from build123d import *

# Parameters (mm, degrees)
F1_DEPTH  = 64
F3_D      = 12
F5_DEPTH  = 21
F7_DEPTH  = 8
F9_DEPTH  = 21
F11_DEPTH = 8
F13_DEPTH = 25
F14_D     = 8.5


with BuildPart() as f1:
    # F0 (on Top) → F1 (new body)
    with BuildSketch(Plane.XY):
        Polygon((-65, 0), (-1.9, 0), (0, -2), (0, 20), (-70.3589838486, 20), align=None)
    extrude(amount=F1_DEPTH)

    # F3 (through all)
    with Locations(Plane(origin=(-60.645825623, -16.25, 0), x_dir=(0.2588190451, -0.9659258263, 0), z_dir=(-0.9659258263, -0.2588190451, 0))):
        with Locations((-24.5287615399, 48), (-24.5287615399, 16)):
            Hole(F3_D / 2)

    # F4 (on face) → F5 (join)
    with BuildSketch(Plane(origin=(0, 0, 0), x_dir=(1, 0, 0), z_dir=(0, 0, -1))):
        Polygon((-35, -20), (0, -20), (0, 0), (-1.9, 0), (-35, 0), align=None)
        Polygon((-1.9, 0), (0, 0), (0, 2), align=None)
    extrude(amount=F5_DEPTH)

    # F6 (on face) → F7 (cut)
    with BuildSketch(Plane(origin=(0, 20, 0), x_dir=(-1, 0, 0), z_dir=(0, 1, 0))):
        Polygon((25.897114317, -17.25), (29.7942286341, -10.5), (22, -10.5), (22, -17.25), align=None)
        Polygon((22, -10.5), (29.7942286341, -10.5), (25.897114317, -3.75), (18.102885683, -3.75), (14.2057713659, -10.5), align=None)
        Polygon((22, -17.25), (22, -10.5), (14.2057713659, -10.5), (18.102885683, -17.25), align=None)
    extrude(amount=-F7_DEPTH, mode=Mode.SUBTRACT)

    # F8 (on face) → F9 (join)
    with BuildSketch(Plane.XY.offset(64)):
        Polygon((0, 0), (0, 20), (-35, 20), (-35, 0), (-1.9, 0), align=None)
        Polygon((0, -2), (0, 0), (-1.9, 0), align=None)
    extrude(amount=F9_DEPTH)

    # F10 (on face) → F11 (cut)
    with BuildSketch(Plane(origin=(0, 20, 0), x_dir=(-1, 0, 0), z_dir=(0, 1, 0))):
        Polygon((25.7527767497, 68), (29.5055534995, 74.5), (14.4944465005, 74.5), (18.2472232503, 68), align=None)
        Polygon((14.4944465005, 74.5), (29.5055534995, 74.5), (25.7527767497, 81), (18.2472232503, 81), align=None)
    extrude(amount=-F11_DEPTH, mode=Mode.SUBTRACT)

    # F12 (on face) → F13 (cut)
    with BuildSketch(Plane(origin=(0, 12, 0), x_dir=(-1, 0, 0), z_dir=(0, 1, 0))):
        with BuildLine():
            Line((19.875, 70.8193920339), (24.125, 78.1806079661))
            ThreePointArc((24.125, 78.1806079661), (18.3193920339, 76.625), (19.875, 70.8193920339))
        make_face()
        with BuildLine():
            ThreePointArc((26.25, 74.5), (25.6806079661, 76.625), (24.125, 78.1806079661))
            Line((24.125, 78.1806079661), (19.875, 70.8193920339))
            ThreePointArc((19.875, 70.8193920339), (24.125, 70.8193920339), (26.25, 74.5))
        make_face()
    extrude(amount=-F13_DEPTH, mode=Mode.SUBTRACT)

    # F14 (through all)
    with Locations(Plane(origin=(0, 20, 0), x_dir=(-1, 0, 0), z_dir=(0, 1, 0))):
        with Locations((22, -10.5)):
            Hole(F14_D / 2)


solid = f1.part
Verification items for the finished model (mm, model axes). A direction names the side the tool comes from. Coordinates: 2 decimals unless noted, no trailing zeros. Order: outer loops, then holes, each group sorted by start corner. A loop starts at its lowest first (then second) coordinate and runs counter-clockwise, first axis right, second up. Notation, with made-up numbers: M 83,26 L 91,26 A20 ccw 91,43 Z; hole C -33.5,-12 d1. An arc over 180 degrees is marked long. One line per item, written item: value. Start each with the question number.
Item 1: Mould release check, pull along Z, two halves, no side actions. Record for faces 4 (the cylindrical face through (-25.37, 5.92, -13.09)), 5 (the flat face through (-18, 12, 85)), 6 (the flat face through (-35, 10, -10)): pulls with the +Z half, pulls with the -Z half, needs draft (parallel to the pull), parting line crosses it, or undercut.
Item 2: Access from +Z, -Z, +X, -X, +Y, -Y to the whole of each face (thin tool, end or side, straight path). Record for faces 1 (the flat face through (-27, 0, 31)), 2 (the flat face through (-27.6, 16.1, 71.2)), 3 (the cylindrical face through (-39.454, 8.617, 16.264)).
Item 3: Thickness scan on probe 1 along Z at (x, y) = (-22, 4.25); probe 2 along Z at (x, y) = (-21, 12.25); probe 3 along Z at (x, y) = (-27.5, 15.5). Record the ranges inside material, lowest first.
Item 4: Sectioned sample at B-B on x = -22. Give the number of separate pieces and of enclosed holes in the cut face, then the cut area to 3 significant figures.
Item 5: Sectioned sample at A-A on z = 43.5. Record the cut outline in (x, y).
Item 6: Depth check by flat-ended pin: P1, Ø19, axis at x = -46.5, z = 29.5, coming from the -Y side; P2, Ø2, axis at x = -38.5, y = 5, coming from the +Z side; P3, Ø11, axis at x = -22, z = -10.5, coming from the +Y side. Enter the tip coordinate at first touch or a pass-through.
Calculated:
1. face 4: undercut
1. face 5: pulls with the +Z half
1. face 6: needs draft
2. face 1: +Z, -Z, -X, -Y
2. face 2: +Y
2. face 3: none
3. probe 1: -21 to -14.75, -6.25 to 70.25, 78.75 to 85
3. probe 2: -21 to -17.25, -3.75 to 68, 81 to 85
3. probe 3: -21 to -14.47, -6.53 to 10.52, 21.48 to 42.52, 53.48 to 71.03, 77.97 to 85
4. separate pieces: 3
4. enclosed holes: 0
4. area: 1,570 mm^2
5. outline: M -70.36,20 L -68.02,11.28 L -35.46,20 Z; M -65.97,3.61 L -65,0 L -1.9,0 L 0,-2 L 0,20 L -4.8,20 Z
6. P1: y = 0
6. P2: z = 64
6. P3: y = 12
